Autodesk Inventor part; units mm, degrees
ref_plane "Work Plane1" through (34.0098, 33.0258, 0) normal (0.866, -0.5, 0) x (0, 0, 1)
ref_plane "YZ Plane" through (0, 0, 0) normal (1, 0, 0) x (0, 1, 0)
ref_plane "XZ Plane" through (0, 0, 0) normal (0, 1, 0) x (-1, 0, 0)
sketch "Sketch1" plane through (0, 0, 0) normal (0, 0, 1) x (1, 0, 0)
  circle A0 centre (34.0098, 33.0258) radius 5
  circle A1 centre (34.0098, 33.0258) radius 8.425
  line L0 (38.874, 41.4508) -> (43.7382, 33.0258)
  line L1 (43.7382, 33.0258) -> (38.874, 24.6008)
  line L2 (38.874, 24.6008) -> (29.1457, 24.6008)
  line L3 (29.1457, 24.6008) -> (24.2815, 33.0258)
  line L4 (24.2815, 33.0258) -> (29.1457, 41.4508)
  line L5 (29.1457, 41.4508) -> (38.874, 41.4508)
  point P0 (34.0098, 41.4508)
  dimension "d1" = 16.85
  dimension "d0" = 10
extrude "Extrusion1" add sketch "Sketch1" along normal blind 8
ref_plane "Work Plane1" through (34.0098, 33.0258, 0) normal (0.866, -0.5, 0) x (0, 0, 1)
thread "Thread1"
sketch "Sketch4" plane through (0, 0, 8) normal (0, 0, 1) x (1, 0, 0)
  circle A0 centre (34.0098, 33.0258) radius 5
  circle A1 centre (34.0098, 33.0258) radius 8.25
  circle A2 centre (34.0098, 33.0258) radius 5.1
  dimension "d11" = 16.5
  dimension "d12" = 10.2
extrude "Extrusion2" add sketch "Sketch4" along normal blind 1.7 contours A1
fillet "Fillet1" radius 0.5 2 edges at (28.9098, 33.0258, 9.7) (25.7598, 33.0258, 9.7)
properties part number "M10 Nut (o'ring)"
The listing builds one solid part. Answer for the finished solid, in the listing's coordinates (mm). A direction names the side the tool comes from. Give positions to 0.01 mm unless a question says otherwise; leave off trailing zeros. Order: outer loops, then holes, each group sorted by start corner. A loop starts at its lowest first (then second) coordinate and runs counter-clockwise, first axis right, second up.
1) Find section B-B on z = 8.5. Write down the section's boundary in (x, y).
Reported:
outline: circle Ø16.5 at (34.01, 33.03); hole circle Ø10.2 at (34.01, 33.03)
2) Determine the mould class of faces 1 (the face through (32.9, 37.9, 3.9)), 2 (the face through (26.68, 37.18, 3.94)), 3 (the face through (34, 24.601, 4)) for opening direction X: pulls with the +X half, pulls with the -X half, needs draft (parallel to the pull), parting line crosses it, or undercut.
Reported:
face 1: undercut
face 2: pulls with the -X half
face 3: needs draft
3) Consider line 1 along Z through (x, y) = (28.5, 32.5); line 2 along Y through (x, z) = (30.25, 7.25); line 3 along Y through (x, z) = (38, 7.75). Determine where each line is inside the solid, lowest interval first.
Reported:
line 1: z = 0 to 9.7
line 2: y = 24.6 to 29.73, 36.32 to 41.45
line 3: y = 24.6 to 30.01, 36.04 to 41.45
4) For faces 4 (the face through (43, 33, 8)), 5 (the face through (34, 41.451, 4)), determine the directions among +Z, -Z, +X, -X, +Y, -Y from which every point of the face is accessible in a straight line to the end or side of a thin tool.
Reported:
face 4: +Z
face 5: +Z, -Z, +X, -X, +Y
5) Given P1, Ø2, axis at y = 29, z = 2, coming from the -X side; P2, Ø1.5, axis at x = 27.5, z = 2.5, coming from the -Y side, each flat-ended and moving along its own axis, determine where each tip first touches the part or whether it passes through.
Reported:
P1: stops at x = 26.03
P2: stops at y = 26.15
6) Find section A-A on z = 5. Write down the section's boundary in (x, y).
Reported:
outline: (24.28, 33.03) - (29.15, 24.6) - (38.87, 24.6) - (43.74, 33.03) - (38.87, 41.45) - (29.15, 41.45) - close; hole circle Ø10 at (34.01, 33.03)
